Design review of the part built by this model. Coordinates are the model's own, in mm. A direction names the side the tool comes from. Give positions to 0.01 mm unless a question says otherwise; leave off trailing zeros. Loops run counter-clockwise (first coordinate to the right, second up) from the corner with the lowest first, then second, coordinate; pieces in that order, holes last. Notation, with made-up numbers: (25.25, 67) - (71.25, 67) arc R21 cw to (71.25, 96) - close; hole circle Ø3 at (-12, 85.5). An arc over 180 degrees is marked (long way). Write each question's results on one line, items separated by ' | '.
```python
from build123d import *

# Parameters (mm, degrees)
SALIENTE_EXTRUIR1_DEPTH = 20
CROQUIS2_R              = 4
CORTAR_EXTRUIR1_DEPTH   = 1.2
CROQUIS3_R              = 1
CORTAR_EXTRUIR2_DEPTH   = 1.8
CROQUIS5_R              = 1
SALIENTE_EXTRUIR2_DEPTH = 1


with BuildPart() as part:
    # Croquis1 → Saliente-Extruir1 (new body)
    with BuildSketch(Plane(origin=(0, 0, 0), x_dir=(1, 0, 0), z_dir=(0, 1, 0))):
        Polygon((3.21663979, -38.197597505), (3.21663979, 11.802402495), (33.21663979, 11.802402495), (33.21663979, 14.802402495), (-29.78336021, 14.802402495), (-29.78336021, 11.802402495), (0.21663979, 11.802402495), (0.21663979, -38.197597505), align=None)
    extrude(amount=SALIENTE_EXTRUIR1_DEPTH)

    # Croquis2 → Cortar-Extruir1 (cut)
    with BuildSketch(Plane(origin=(3.21663979, 0, 0), x_dir=(0, 0, -1), z_dir=(1, 0, 0))):
        with Locations((-18.197597505, 10)):
            Circle(CROQUIS2_R)
    extrude(amount=-CORTAR_EXTRUIR1_DEPTH, mode=Mode.SUBTRACT)

    # Croquis3 → Cortar-Extruir2 (cut)
    with BuildSketch(Plane(origin=(2.01663979, 0, 0), x_dir=(0, 0, -1), z_dir=(1, 0, 0))):
        with Locations((-18.197597505, 10)):
            Circle(CROQUIS3_R)
    extrude(amount=-CORTAR_EXTRUIR2_DEPTH, mode=Mode.SUBTRACT)

    # Croquis5 → Saliente-Extruir2 (add)
    with BuildSketch(Plane(origin=(0, 0, -14.802402495), x_dir=(-1, 0, 0), z_dir=(0, 0, -1))):
        with Locations(Location((-1.71663979, 10, 0), (0, 0, 180))):
            Circle(CROQUIS5_R)
    extrude(amount=SALIENTE_EXTRUIR2_DEPTH)


solid = part.part
```
Item 1: Clearance check with flat-ended pins moving along their axes: P1, Ø12, axis at x = -8, y = 9, coming from the +Z side; P2, Ø4, axis at y = 11.5, z = 13, coming from the -X side; P3, Ø6.5, axis at y = 10, z = 18.2, coming from the +X side. State where each tip first meets the part, or that it passes through.
Output values:
P1: stops at z = -11.8 | P2: stops at x = 0.22 | P3: stops at x = 2.02
Item 2: Tool access review of faces 1 (the face through (-15, 10, -11.802)), 2 (the face through (1.59, 9.01, -15.3)), 3 (the face through (2.625, 10.176, 22.194)), 4 (the face through (-29.783, 10, -13)), 5 (the face through (18, 10, -11.802)): name each direction out of +Z, -Z, +X, -X, +Y, -Y from which nothing blocks a thin tool from reaching the whole face with its end or side.
Output values:
face 1: +Z, -X, +Y, -Y | face 2: -Z | face 3: +X | face 4: +Z, -Z, -X, +Y, -Y | face 5: +Z, +X, +Y, -Y
Item 3: We need section B-B on y = 2.5. Give the boundary of the cut face in (x, z), then the cut area to 3 significant figures.
Output values:
outline: (-29.78, -14.8) - (33.22, -14.8) - (33.22, -11.8) - (3.22, -11.8) - (3.22, 38.2) - (0.22, 38.2) - (0.22, -11.8) - (-29.78, -11.8) - close | area: 339 mm²
Item 4: Wall thickness on probe 1 along X at (y, z) = (8, 30.5); probe 2 along Z at (x, y) = (30.5, 8.75): over which ranges is each line inside the solid? List them lowest first.
Output values:
probe 1: x = 0.22 to 3.22 | probe 2: z = -14.8 to -11.8
Item 5: Draft analysis for pull direction Y (two halves, no side actions). For faces 6 (the face through (1.129, 10.3, 17.244)), 7 (the face through (2, 20, -4)), 8 (the face through (2, 12, -14.802)), 9 (the face through (2.017, 9, 17)), state which applies: +Y half, -Y half, draft (parallel to the pull), parting line (faces both ways), or undercut.
Output values:
face 6: undercut | face 7: +Y half | face 8: draft | face 9: undercut
Item 6: We need section C-C on z = -8. Give the boundary of the cut face in (x, y).
Output values:
outline: (0.22, 0) - (3.22, 0) - (3.22, 20) - (0.22, 20) - close
Item 7: We need section D-D on x = -4.5. Give the boundary of the cut face in (y, z), then the cut area to 3 significant figures.
Output values:
outline: (0, -14.8) - (20, -14.8) - (20, -11.8) - (0, -11.8) - close | area: 60.0 mm²
Item 8: We need section A-A on y = 10. Give the boundary of the cut face in (x, z), then the cut area to 3 significant figures.
Output values:
outline: (-29.78, -14.8) - (0.72, -14.8) - (0.72, -15.8) - (2.72, -15.8) - (2.72, -14.8) - (33.22, -14.8) - (33.22, -11.8) - (3.22, -11.8) - (3.22, 14.2) - (2.02, 14.2) - (2.02, 17.2) - (0.22, 17.2) - (0.22, -11.8) - (-29.78, -11.8) - close; (0.22, 19.2) - (2.02, 19.2) - (2.02, 22.2) - (3.22, 22.2) - (3.22, 38.2) - (0.22, 38.2) - close | area: 328 mm²
